Can you work these out from the drawing? Everything is in mm from the part's minimum corner. A direction names the side the tool comes from. Round coordinates to 2 decimals unless told otherwise and drop trailing zeros. Loops run counter-clockwise (first coordinate to the right, second up) from the corner with the lowest first, then second, coordinate; pieces in that order, holes last. Notation, with made-up numbers: (36.25, 56.5) - (52.25, 56.5) arc R35 ccw to (52.25, 91.5) - close; hole circle Ø5 at (53, -12). An arc over 180 degrees is marked (long way). Answer as a JSON object with one key per item and string values. Group by question number.
1) Which directions (+Z, -Z, +X, -X, +Y, -Y) give clear straight access to the entire face, cutting with the end or side of a thin tool? Please do the marked faces 1, 2 and 3.
2) I want a section at A-A, the plane y = 25. Please give me the cut outline in (x, z), then the cut area to 3 significant figures.
3) Will these pins go through, and if not, where does the flat tip stop? P1, Ø1.5, axis at y = 4, z = 163.5, coming from the +X side; P2, Ø2, axis at x = 166, z = 82.5, coming from the -Y side (1 decimal); P3, Ø3, axis at x = 197, z = 137, coming from the -Y side; P4, Ø7, axis at x = 94, y = 20, coming from the +Z side.
4) If I drill on line 1 along Z through (x, y) = (42, 25.25); line 2 along Z through (x, y) = (160.5, 19.5); line 3 along Z through (x, y) = (43.5, 21.25), over which ranges is the centre line in solid material (lowest first)? Write a range as [from, to].
5) I want a section at B-B, the plane x = 172. Please give me the cut outline in (y, z) (1 decimal), then the cut area to 3 significant figures.
6) I want a section at D-D, the plane x = 34. Please give me the cut outline in (y, z) (1 decimal).
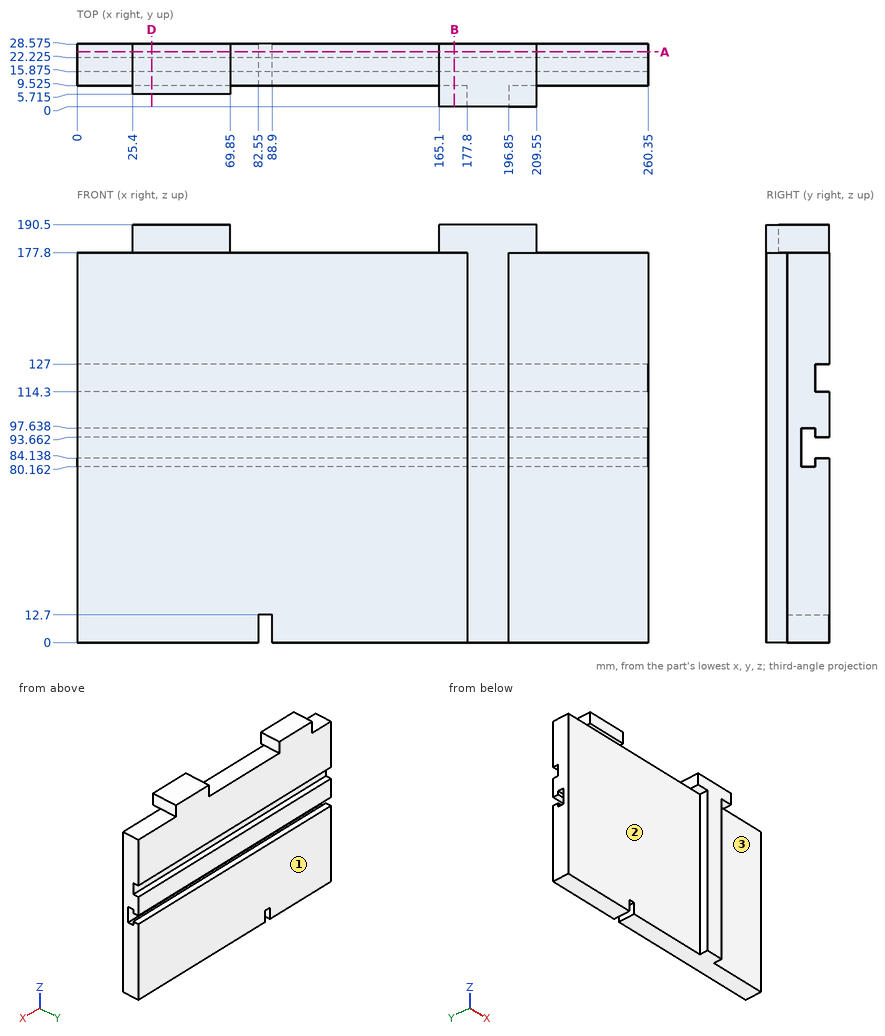
Outcome:
{
 "1": {"face 1": "+Z, -Z, +X, -X, +Y", "face 2": "-Z, -X, -Y", "face 3": "-Z, +X, -Y"},
 "2": {"outline": "(0, 0) - (82.55, 0) - (82.55, 12.7) - (88.9, 12.7) - (88.9, 0) - (260.35, 0) - (260.35, 84.14) - (0, 84.14) - close; (0, 93.66) - (260.35, 93.66) - (260.35, 114.3) - (0, 114.3) - close; (0, 127) - (260.35, 127) - (260.35, 177.8) - (209.55, 177.8) - (209.55, 190.5) - (165.1, 190.5) - (165.1, 177.8) - (69.85, 177.8) - (69.85, 190.5) - (25.4, 190.5) - (25.4, 177.8) - (0, 177.8) - close", "area": "41,600 mm^2"},
 "3": {"P1": "x = 196.85", "P2": "y = 9.5", "P3": "y = 0", "P4": "z = 177.8"},
 "4": {"line 1": "[0, 84.14], [93.66, 114.3], [127, 190.5]", "line 2": "[0, 80.16], [97.64, 177.8]", "line 3": "[0, 80.16], [97.64, 190.5]"},
 "5": {"outline": "(0, 177.8) - (9.5, 177.8) - (9.5, 0) - (28.6, 0) - (28.6, 84.1) - (22.2, 84.1) - (22.2, 80.2) - (15.9, 80.2) - (15.9, 97.6) - (22.2, 97.6) - (22.2, 93.7) - (28.6, 93.7) - (28.6, 114.3) - (22.2, 114.3) - (22.2, 127) - (28.6, 127) - (28.6, 190.5) - (0, 190.5) - close", "area": "3,500 mm^2"},
 "6": {"outline": "(5.7, 177.8) - (9.5, 177.8) - (9.5, 0) - (28.6, 0) - (28.6, 84.1) - (22.2, 84.1) - (22.2, 80.2) - (15.9, 80.2) - (15.9, 97.6) - (22.2, 97.6) - (22.2, 93.7) - (28.6, 93.7) - (28.6, 114.3) - (22.2, 114.3) - (22.2, 127) - (28.6, 127) - (28.6, 190.5) - (5.7, 190.5) - close"}
}
